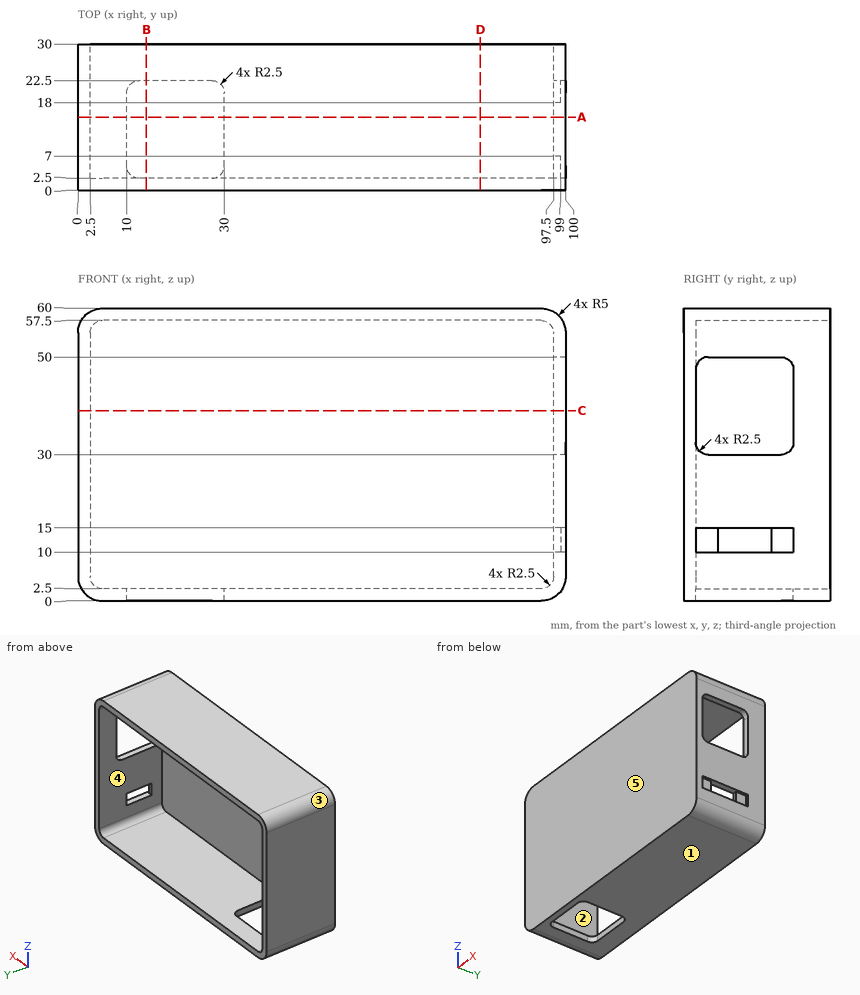
Drawing for the job (mm, zero at the part's lowest x, y, z). A direction names the side the tool comes from. Coordinates: 2 decimals unless noted, no trailing zeros. Order: outer loops, then holes, each group sorted by start corner. A loop starts at its lowest first (then second) coordinate and runs counter-clockwise, first axis right, second up. Notation, with made-up numbers: (53, 34) -> (78, 34) arc R22 ccw to (78, 46) -> close; hole circle Ø11 at (8, -36). An arc over 180 degrees is marked (long way). Return JSON: item names as keys, results as strings.
Item 1: Slice it at A-A (y = 15). Write the cut outline in (x, z).
Model answer:
{"outline": "(0, 5) arc R5 ccw to (5, 0) -> (10, 0) -> (10, 2.5) -> (5, 2.5) arc R2.5 cw to (2.5, 5) -> (2.5, 55) arc R2.5 cw to (5, 57.5) -> (95, 57.5) arc R2.5 cw to (97.5, 55) -> (97.5, 50) -> (100, 50) -> (100, 55) arc R5 ccw to (95, 60) -> (5, 60) arc R5 ccw to (0, 55) -> close; (30, 0) -> (95, 0) arc R5 ccw to (100, 5) -> (100, 10) -> (97.5, 10) -> (97.5, 5) arc R2.5 cw to (95, 2.5) -> (30, 2.5) -> close; (97.5, 15) -> (100, 15) -> (100, 30) -> (97.5, 30) -> close"}
Item 2: 3-axis set-ups, long thin cutter, end or side, ignore diameter. For the marked faces 1 and 2: which of +Z, -Z, +X, -X, +Y, -Y reach the whole face in a straight line?
Model answer:
{"face 1": "-Z, +X, -X, +Y, -Y", "face 2": "+Y"}
Item 3: Slice it at B-B (x = 14). Write the cut outline in (y, z).
Model answer:
{"outline": "(0, 0) -> (2.5, 0) -> (2.5, 57.5) -> (30, 57.5) -> (30, 60) -> (0, 60) -> close; (22.5, 0) -> (30, 0) -> (30, 2.5) -> (22.5, 2.5) -> close"}
Item 4: Slice it at D-D (x = 82.5). Write the cut outline in (y, z), then the cut area to 4 significant figures.
Model answer:
{"outline": "(0, 0) -> (30, 0) -> (30, 2.5) -> (2.5, 2.5) -> (2.5, 57.5) -> (30, 57.5) -> (30, 60) -> (0, 60) -> close", "area": "287.5 mm²"}
Item 5: Mould opens along Z. For the marked faces 3, 4 and 5 say: pulls with the +Z half, pulls with the -Z half, needs draft (parallel to the pull), parting line crosses it, or undercut.
Model answer:
{"face 3": "pulls with the +Z half", "face 4": "undercut", "face 5": "needs draft"}
Item 6: Slice it at C-C (z = 39). Write the cut outline in (x, y).
Model answer:
{"outline": "(0, 0) -> (100, 0) -> (100, 2.5) -> (2.5, 2.5) -> (2.5, 30) -> (0, 30) -> close; (97.5, 22.5) -> (100, 22.5) -> (100, 30) -> (97.5, 30) -> close"}
Item 7: Pin check, flat tips, straight feed: P1, Ø1.3, axis at y = 21, z = 12.5, coming from the +X side; P2, Ø0.8, axis at x = 98.5, y = 12.5, coming from the +Z side; P3, Ø3, axis at x = 99, y = 9, coming from the -Z side. Stop position of each tip, or through.
Model answer:
{"P1": "stops at x = 99", "P2": "stops at z = 58.92", "P3": "stops at z = 0.67"}
Item 8: Wall check: line 1 along X through (y, z) = (16, 28); line 2 along X through (y, z) = (5.25, 14); line 3 along Z through (x, y) = (51.5, 21.5). Give the ranges that are in metal, low to high. Write a range as from..to.
Model answer:
{"line 1": "x = 0..2.5, 97.5..100", "line 2": "x = 0..2.5, 97.5..99", "line 3": "z = 0..2.5, 57.5..60"}
